from build123d import *

# Parameters (mm, degrees)
SKETCH1_W           = 90
SKETCH1_H           = 60
BOSS_EXTRUDE1_DEPTH = 2
SKETCH2_R           = 2.5
CUT_EXTRUDE1_DEPTH  = 10
SKETCH3_W           = 2
SKETCH3_H           = 60
BOSS_EXTRUDE4_DEPTH = 27.5
SKETCH4_W           = 20
SKETCH4_H           = 40.5
CUT_EXTRUDE2_DEPTH  = 10


with BuildPart() as part:
    # Sketch1 → Boss-Extrude1 (new body)
    with BuildSketch(Plane.XY):
        Rectangle(SKETCH1_W, SKETCH1_H)
    extrude(amount=BOSS_EXTRUDE1_DEPTH)

    # Sketch2 → Cut-Extrude1 (cut)
    with BuildSketch(Plane.XY.offset(2)):
        with Locations((-40, -25)):
            Circle(SKETCH2_R)
        with Locations((-40, 25)):
            Circle(SKETCH2_R)
        with Locations((40, 25)):
            Circle(SKETCH2_R)
        with Locations((40, -25)):
            Circle(SKETCH2_R)
    extrude(amount=-CUT_EXTRUDE1_DEPTH, mode=Mode.SUBTRACT)

    # Sketch3 → Boss-Extrude4 (add)
    with BuildSketch(Plane(origin=(0, 0, 0), x_dir=(-1, 0, 0), z_dir=(0, 0, -1))):
        with Locations((-36, 0)):
            Rectangle(SKETCH3_W, SKETCH3_H)
    extrude(amount=BOSS_EXTRUDE4_DEPTH)

    # Sketch4 → Cut-Extrude2 (cut)
    with BuildSketch(Plane(origin=(37, 0, 0), x_dir=(0, 0, -1), z_dir=(1, 0, 0))):
        with Locations((17.5, -1.75)):
            Rectangle(SKETCH4_W, SKETCH4_H)
    extrude(amount=-CUT_EXTRUDE2_DEPTH, mode=Mode.SUBTRACT)


solid = part.part
Geometry check sheet. Reference: the model listing, model coordinates, mm. A direction names the side the tool comes from. Round coordinates to 2 decimals unless told otherwise and drop trailing zeros. Write each loop counter-clockwise with the first axis right and the second up, starting at its lowest first coordinate (ties: lowest second). Pieces come first, ordered by that corner, then holes.
Item 1: Section check C-C (y = -25). Record the boundary of the cut face in (x, z).
Determined:
outline: (-45, 0) - (-42.5, 0) - (-42.5, 2) - (-45, 2) - close; (-37.5, 0) - (35, 0) - (35, -27.5) - (37, -27.5) - (37, 0) - (37.5, 0) - (37.5, 2) - (-37.5, 2) - close; (42.5, 0) - (45, 0) - (45, 2) - (42.5, 2) - close
Item 2: Material ranges on line 1 along Y through (x, z) = (40, 0.8); line 2 along Z through (x, y) = (3.5, -18); line 3 along X through (y, z) = (19, -18.5), recorded low to high.
Determined:
line 1: y = -30 to -27.5, -22.5 to 22.5, 27.5 to 30
line 2: z = 0 to 2
line 3: x = 35 to 37
Item 3: Access from +Z, -Z, +X, -X, +Y, -Y to the whole of each face (thin tool, end or side, straight path). Record for faces 1 (the face through (35, 0, -7)), 2 (the face through (37, 0, -7)), 3 (the face through (36, -22, -17)).
Determined:
face 1: -Z, -X, +Y, -Y
face 2: -Z, +X, +Y, -Y
face 3: -Z, +X, -X
Item 4: Section check B-B (x = -40). Record the boundary of the cut face in (y, z), plus the area to 3 significant figures.
Determined:
outline: (-30, 0) - (-27.5, 0) - (-27.5, 2) - (-30, 2) - close; (-22.5, 0) - (22.5, 0) - (22.5, 2) - (-22.5, 2) - close; (27.5, 0) - (30, 0) - (30, 2) - (27.5, 2) - close
area: 100 mm2
Item 5: Section check D-D (y = 10.5). Record the boundary of the cut face in (x, z), plus the area to 3 significant figures.
Determined:
outline: (-45, 0) - (35, 0) - (35, -7.5) - (37, -7.5) - (37, 0) - (45, 0) - (45, 2) - (-45, 2) - close
area: 195 mm2
Item 6: Mould release check, pull along Y, two halves, no side actions. Record for faces 4 (the face through (36, -2, -7.5)), 5 (the face through (9.8, 30, 0.3)), 6 (the face through (36, 24, -27.5)): +Y half, -Y half, draft (parallel to the pull), parting line (faces both ways), or undercut.
Determined:
face 4: undercut
face 5: +Y half
face 6: draft
Item 7: Go/stop test with flat-tipped pins: pin 1 Ø4 at (x, y) = (-29.5, 12.5) entering from -Z; pin 2 Ø8 at (y, z) = (8, -8) entering from -X; pin 3 Ø9 at (x, y) = (40, 5) entering from -Z. Record where each tip stops, or that it passes through.
Determined:
pin 1: stops at z = 0
pin 2: stops at x = 35
pin 3: stops at z = -7.5
Item 8: Section check A-A (z = -12). Record the boundary of the cut face in (x, y), plus the area to 3 significant figures.
Determined:
outline: (35, -30) - (37, -30) - (37, -22) - (35, -22) - close; (35, 18.5) - (37, 18.5) - (37, 30) - (35, 30) - close
area: 39.0 mm2
